from build123d import *

# Parameters (mm, degrees)
SKETCH1_W           = 5
SKETCH1_H           = 80
BOSS_EXTRUDE1_DEPTH = 2
SKETCH3_R           = 0.95
CUT_EXTRUDE1_DEPTH  = 41.127920454
SKETCH2_W           = 2
SKETCH2_H           = 8
BOSS_EXTRUDE2_DEPTH = 6
CUT_EXTRUDE2_REACH  = 50.5
SKETCH4_R           = 1.1
CHAMFER1_SIZE       = 5
CHAMFER2_SIZE       = 1


with BuildPart() as part:
    # Sketch1 → Boss-Extrude1 (new body)
    with BuildSketch(Plane.XY):
        Rectangle(SKETCH1_W, SKETCH1_H)
    extrude(amount=BOSS_EXTRUDE1_DEPTH)

    # Sketch3 → Cut-Extrude1 (cut, through all)
    with BuildSketch(Plane.XY.offset(2)):
        with Locations((0, 35)):
            Circle(SKETCH3_R)
        with Locations((0, 30)):
            Circle(SKETCH3_R)
        with Locations((0, 25)):
            Circle(SKETCH3_R)
        with Locations((0, 20)):
            Circle(SKETCH3_R)
        with Locations((0, 15)):
            Circle(SKETCH3_R)
        with Locations((0, 10)):
            Circle(SKETCH3_R)
        with Locations((0, 5)):
            Circle(SKETCH3_R)
        Circle(SKETCH3_R)
        with Locations((0, -5)):
            Circle(SKETCH3_R)
        with Locations((0, -10)):
            Circle(SKETCH3_R)
        with Locations((0, -15)):
            Circle(SKETCH3_R)
        with Locations((0, -20)):
            Circle(SKETCH3_R)
        with Locations((0, -25)):
            Circle(SKETCH3_R)
        with Locations((0, -30)):
            Circle(SKETCH3_R)
    extrude(amount=-CUT_EXTRUDE1_DEPTH, mode=Mode.SUBTRACT)

    # Sketch2 → Boss-Extrude2 (add)
    with BuildSketch(Plane(origin=(0, 0, 0), x_dir=(-1, 0, 0), z_dir=(0, 0, -1))):
        with Locations((0, -44)):
            Rectangle(SKETCH2_W, SKETCH2_H)
    extrude(amount=-BOSS_EXTRUDE2_DEPTH)

    # Sketch4 → Cut-Extrude2 (cut, up to next)
    with BuildSketch(Plane.ZY.offset(1), mode=Mode.PRIVATE) as cut_extrude2_sk1:
        with Locations((3, -44)):
            Circle(SKETCH4_R)
    cut_extrude2_tool1 = extrude(cut_extrude2_sk1.sketch, amount=-CUT_EXTRUDE2_REACH, mode=Mode.PRIVATE) & part.part
    # Sketch4 → Cut-Extrude2 (cut, up to next)
    with BuildSketch(Plane.ZY.offset(1), mode=Mode.PRIVATE) as cut_extrude2_sk2:
        with BuildLine():
            Line((0, -45.802775638), (0, -48))
            Line((0, -48), (6, -48))
            Line((6, -48), (6, -45.802775638))
            ThreePointArc((6, -45.802775638), (3, -47.5), (0, -45.802775638))
        make_face()
    cut_extrude2_tool2 = extrude(cut_extrude2_sk2.sketch, amount=-CUT_EXTRUDE2_REACH, mode=Mode.PRIVATE) & part.part
    add(cut_extrude2_tool1.solids().sort_by_distance((-1, -44, 3))[0], mode=Mode.SUBTRACT)
    add(cut_extrude2_tool2.solids().sort_by_distance((-1, -47.563897, 3))[0], mode=Mode.SUBTRACT)

    # Chamfer1
    # the kernel refuses this chamfer: 5 mm, written as the material it adds along each edge
    with BuildSketch(Plane(origin=(-1, -40, 2), x_dir=(0, 0.9996219169112968, -0.02749587661058636), z_dir=(1, 0, 0))) as chamfer1_piece_1_section:
        Polygon((CHAMFER1_SIZE * 0.999621916911, CHAMFER1_SIZE * 0.0274958766106), (-CHAMFER1_SIZE * 0.0274958766106, CHAMFER1_SIZE * 0.999621916911), (0, 0), align=None)
    chamfer1_piece_1 = extrude(amount=2, mode=Mode.PRIVATE)
    chamfer1_piece_1 = split(chamfer1_piece_1, bisect_by=Plane(origin=(0, -38.277777778, 6), z_dir=(0, 0, -1)), keep=Keep.TOP, mode=Mode.PRIVATE)
    add(chamfer1_piece_1)

    # Chamfer2
    chamfer2_edges = [part.edges().sort_by_distance(p)[0] for p in [
        (-2.5, 40, 1),
        (2.5, 40, 1),
        (-2.5, -40, 1),
        (2.5, -40, 1),
    ]]
    chamfer(chamfer2_edges, length=CHAMFER2_SIZE)


solid = part.part
Part model, mm, in its own coordinate system. Round coordinates to 2 decimals unless told otherwise and drop trailing zeros. Loops run counter-clockwise (first coordinate to the right, second up) from the corner with the lowest first, then second, coordinate; pieces in that order, holes last. Notation, with made-up numbers: (84.25, -32) - (102.25, -32) arc R9 ccw to (102.25, -17) - close; hole circle Ø9 at (58, -12). An arc over 180 degrees is marked (long way). Answer as a JSON object with one key per item and string values.
Item 1: Pin check, flat tips, straight feed: pin 1 (1.1 mm diameter, centred on x = 0, y = 10, fed in from +Z); pin 2 (3 mm diameter, centred on x = 0, y = -5, fed in from +Z); pin 3 (2 mm diameter, centred on x = 0, y = 15, fed in from -Z); pin 4 (0.6 mm diameter, centred on x = -1.5, z = 1, fed in from -Y). Stop position of each tip, or through.
Output:
{"pin 1": "through", "pin 2": "z = 2", "pin 3": "z = 0", "pin 4": "y = -40"}
Item 2: Band-saw the part on B-B on z = 2.75. List the corners of the cut face in (x, y), plus the area to 3 significant figures.
Output:
{"outline": "(-1, -47.49) - (1, -47.49) - (1, -45.07) - (-1, -45.07) - close; (-1, -42.93) - (1, -42.93) - (1, -35.75) - (-1, -35.75) - close", "area": "19.2 mm2"}
Item 3: Band-saw the part on D-D on y = 23. List the corners of the cut face in (x, z).
Output:
{"outline": "(-2.5, 0) - (2.5, 0) - (2.5, 2) - (-2.5, 2) - close"}
Item 4: Band-saw the part on A-A on y = -30. List the corners of the cut face in (x, z).
Output:
{"outline": "(-2.5, 0) - (-0.95, 0) - (-0.95, 2) - (-2.5, 2) - close; (0.95, 0) - (2.5, 0) - (2.5, 2) - (0.95, 2) - close"}
Item 5: Band-saw the part on C-C on y = -42. List the corners of the cut face in (x, z), plus the area to 3 significant figures.
Output:
{"outline": "(-1, 0) - (1, 0) - (1, 6) - (-1, 6) - close", "area": "12.0 mm2"}
Item 6: Wall check: L1, parallel to Z at x = -0.15, y = -22; L2, parallel to X at y = -42, z = 5; L3, parallel to Y at x = -0.5, z = 3. Give the ranges that are in metal, low to high.
Output:
{"L1": "0 to 2", "L2": "-1 to 1", "L3": "-47.5 to -45.1, -42.9 to -36"}
Item 7: Pull direction Y, two halves, no side cores. Call faces 1 (the face through (0.44, 4.16, 1.01)), 2 (the face through (-2.5, -1, 1)), 3 (the face through (0, -47.5, 3.1)), 4 (the face through (-0.01, -43.07, 3.59)): pulls with the +Y half, pulls with the -Y half, needs draft (parallel to the pull), parting line crosses it, or undercut.
Output:
{"face 1": "undercut", "face 2": "needs draft", "face 3": "pulls with the -Y half", "face 4": "undercut"}
